Could you check a few things on this model? Use its own coordinates, in mm. A direction names the side the tool comes from. Coordinates: 2 decimals unless noted, no trailing zeros. Write each loop counter-clockwise with the first axis right and the second up, starting at its lowest first coordinate (ties: lowest second). Pieces come first, ordered by that corner, then holes.
Item 1: Which directions (+Z, -Z, +X, -X, +Y, -Y) give clear straight access to the entire face, cutting with the end or side of a thin tool? Please do faces 1 (the flat face through (22.86, 0, -263)), 2 (the flat face through (0, -12.7, -263)).
Item 2: Thinking about a two-plate mould opening in X: for faces 3 (the flat face through (25.4, 0, -263)), 4 (the flat face through (0, 10.16, -263)), 5 (the flat face through (0, 12.7, -263)), 6 (the flat face through (-25.4, 0, -263)), which applies, +X half, -X half, draft (parallel to the pull), parting line (faces both ways), or undercut?
Item 3: I want a section at B-B on z = -122. Please give me the cut outline in (x, y), then the cut area to 3 significant figures.
Item 4: If I drill on probe 1 along Y at (x, z) = (0, -167); probe 2 along X at (y, z) = (3, -350); probe 3 along Y at (x, z) = (24, -292), over which ranges is the centre line in solid material (lowest first)?
Item 5: I want a section at A-A on x = -13.5. Please give me the cut outline in (y, z).
from build123d import *

# Parameters (mm, degrees)
SKETCH1_W             = 50.8
SKETCH1_H             = 25.4
SKETCH1_W_2           = 45.72
SKETCH1_H_2           = 20.32
BOSS_EXTRUDE1_DEPTH   = 533.4
F_8_CLEARANCE_HOLE1_D = 4.4958


with BuildPart() as part:
    # Sketch1 → Boss-Extrude1 (new body)
    with BuildSketch(Plane.XY):
        Rectangle(SKETCH1_W, SKETCH1_H)
        Rectangle(SKETCH1_W_2, SKETCH1_H_2, mode=Mode.SUBTRACT)
    extrude(amount=-BOSS_EXTRUDE1_DEPTH)

    # #8 Clearance Hole1 (through all)
    with Locations(Plane(origin=(25.4, 0, 0), x_dir=(0, 0, -1), z_dir=(1, 0, 0))):
        with Locations((12.7, 0), (38.1, 0), (63.5, 0), (88.9, 0), (114.3, 0), (139.7, 0), (165.1, 0), (190.5, 0), (215.9, 0), (241.3, 0), (266.7, 0), (292.1, 0), (317.5, 0), (342.9, 0), (368.3, 0), (393.7, 0), (419.1, 0), (444.5, 0), (469.9, 0), (495.3, 0), (520.7, 0)):
            Hole(F_8_CLEARANCE_HOLE1_D / 2)


solid = part.part
Response values:
1. face 1: +Z, -Z
1. face 2: +Z, -Z, +X, -X, -Y
2. face 3: +X half
2. face 4: undercut
2. face 5: draft
2. face 6: -X half
3. outline: (-25.4, -12.7) - (25.4, -12.7) - (25.4, 12.7) - (-25.4, 12.7) - close; hole (-22.86, -10.16) - (22.86, -10.16) - (22.86, 10.16) - (-22.86, 10.16) - close
3. area: 361 mm2
4. probe 1: y = -12.7 to -10.16, 10.16 to 12.7
4. probe 2: x = -25.4 to -22.86, 22.86 to 25.4
4. probe 3: y = -12.7 to -2.25, 2.25 to 12.7
5. outline: (-12.7, -533.4) - (-10.16, -533.4) - (-10.16, 0) - (-12.7, 0) - close; (10.16, -533.4) - (12.7, -533.4) - (12.7, 0) - (10.16, 0) - close
